For this review, take the finished solid that the model builds, in its own axes (mm). Round coordinates to 2 decimals unless told otherwise and drop trailing zeros. Order: outer loops, then holes, each group sorted by start corner. A loop starts at its lowest first (then second) coordinate and runs counter-clockwise, first axis right, second up. Notation, with made-up numbers: M 12.25,59 L 63.25,59 A18 cw 63.25,83 Z; hole C 28.5,60.25 d3. An arc over 180 degrees is marked long. Answer as a JSON object with one key per item and string values.
from build123d import *

# Parameters (mm, degrees)
SKETCH1_W            = 90
SKETCH1_H            = 60
BOSS_EXTRUDE1_DEPTH  = 10
SKETCH2_R            = 5
CUT_EXTRUDE1_DEPTH   = 11
LPATTERN1_COUNT      = 4
LPATTERN1_PITCH      = 30
LPATTERN1_COUNT_DIR2 = 4
LPATTERN1_PITCH_DIR2 = 30


with BuildPart() as part:
    # Sketch1 → Boss-Extrude1 (new body)
    with BuildSketch(Plane(origin=(0, 0, 0), x_dir=(1, 0, 0), z_dir=(0, 1, 0))):
        with Locations((45, 30)):
            Rectangle(SKETCH1_W, SKETCH1_H)
    extrude(amount=BOSS_EXTRUDE1_DEPTH)

    # Sketch2 → Cut-Extrude1 (cut, through all)
    with BuildSketch(Plane(origin=(0, 10, 0), x_dir=(1, 0, 0), z_dir=(0, 1, 0))):
        with Locations((15, 15)):
            Circle(SKETCH2_R)
    cut_extrude1 = extrude(amount=-CUT_EXTRUDE1_DEPTH, mode=Mode.SUBTRACT)

    # LPattern1: Cut-Extrude1 4 × 4
    with Locations(*[(i * LPATTERN1_PITCH, 0, -j * LPATTERN1_PITCH_DIR2) for i in range(LPATTERN1_COUNT) for j in range(LPATTERN1_COUNT_DIR2) if (i, j) != (0, 0)]):
        add(cut_extrude1, mode=Mode.SUBTRACT)


solid = part.part
1) Insertion check: P1, Ø6, axis at x = 75, z = -15, coming from the +Y side; P2, Ø4, axis at x = 65.5, z = -53, coming from the -Y side. Each pin has a flat end and moves straight along its axis. Give the tip position at first contact, or say it passes through.
Geometry check:
{"P1": "passes through", "P2": "stops at y = 0"}
2) For L1, parallel to X at y = 2, z = -15; L2, parallel to Z at x = 15, y = 2.75; L3, parallel to Z at x = 48.5, y = 0.5, list the stretches that pass through material, from the lowest coordinate up.
Geometry check:
{"L1": "x = 0 to 10, 20 to 40, 50 to 70, 80 to 90", "L2": "z = -60 to -50, -40 to -20, -10 to 0", "L3": "z = -60 to -48.57, -41.43 to -18.57, -11.43 to 0"}
3) Add section B-B on y = 5.25. State the section outline as (x, z) points.
Geometry check:
{"outline": "M 0,-60 L 90,-60 L 90,0 L 0,0 Z; hole C 15,-45 d10; hole C 15,-15 d10; hole C 45,-45 d10; hole C 45,-15 d10; hole C 75,-45 d10; hole C 75,-15 d10"}
4) Add section C-C on z = -15. State the section outline as (x, y) points, and give its area (3 significant figures).
Geometry check:
{"outline": "M 0,0 L 10,0 L 10,10 L 0,10 Z; M 20,0 L 40,0 L 40,10 L 20,10 Z; M 50,0 L 70,0 L 70,10 L 50,10 Z; M 80,0 L 90,0 L 90,10 L 80,10 Z", "area": "600 mm²"}
5) Add section A-A on x = 45. State the section outline as (y, z) points, and give its area (3 significant figures).
Geometry check:
{"outline": "M 0,-60 L 10,-60 L 10,-50 L 0,-50 Z; M 0,-40 L 10,-40 L 10,-20 L 0,-20 Z; M 0,-10 L 10,-10 L 10,0 L 0,0 Z", "area": "400 mm²"}
6) Mouldability with a two-part tool opening along Z and no side actions: class faces 1 (the cylindrical face through (41, 5, -48)), 2 (the flat face through (44, 0, -30)), 3 (the flat face through (44, 5, -60)) as +Z half, -Z half, draft (parallel to the pull), parting line (faces both ways), or undercut.
Geometry check:
{"face 1": "undercut", "face 2": "draft", "face 3": "-Z half"}
